Check sheet for the drawn part. Datum: minimum x, y, z corner. Units: mm. Coordinates: 2 decimals unless noted, no trailing zeros. Write each loop counter-clockwise with the first axis right and the second up, starting at its lowest first coordinate (ties: lowest second). Pieces come first, ordered by that corner, then holes. Notation, with made-up numbers: (23.25, 52.25) -> (60.25, 52.25) arc R29 cw to (60.25, 72.25) -> close; hole circle Ø7 at (-25.5, 27.25). An arc over 180 degrees is marked (long way). Answer in a Markdown table with one row per item. Add a question column.
1. Cross-section at A-A on z = 6. Record the cut outline in (x, y), and give its area (3 significant figures).
2. Scan lines: L1, parallel to Y at x = 112, z = 6.25; L2, parallel to Y at x = 106, z = 0.75; L3, parallel to X at y = 469.5, z = 2.5. Record each from-to range of solid material in increasing order. Write a range as from..to.
3. Depth check by flat-ended pin: P1, Ø6, axis at y = 536.5, z = 5, coming from the -X side. Enter the tip coordinate at first touch or a pass-through.
4. Cross-section at B-B on x = 115. Record the cut outline in (y, z), and give its area (3 significant figures).
5. Cross-section at C-C on x = 197.5. Record the cut outline in (y, z) (3 decimals), and give its area (3 significant figures).
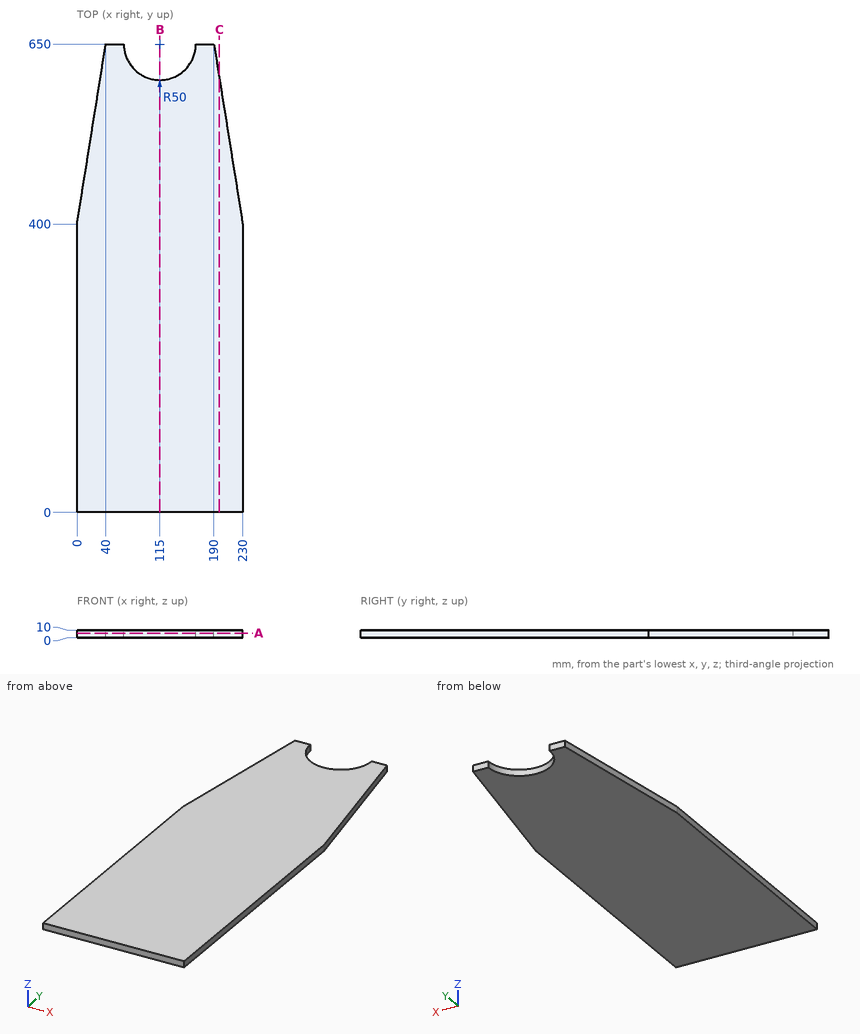
Results found:
| question | item | result |
|---|---|---|
| 1 | outline | (0, 0) -> (230, 0) -> (230, 400) -> (190, 650) -> (165, 650) arc R50 cw to (65, 650) -> (40, 650) -> (0, 400) -> close |
| 1 | area | 136,000 mm^2 |
| 2 | L1 | y = 0..600.09 |
| 2 | L2 | y = 0..600.82 |
| 2 | L3 | x = 11.12..218.88 |
| 3 | P1 | stops at x = 21.36 |
| 4 | outline | (0, 0) -> (600, 0) -> (600, 10) -> (0, 10) -> close |
| 4 | area | 6,000 mm^2 |
| 5 | outline | (0, 0) -> (603.125, 0) -> (603.125, 10) -> (0, 10) -> close |
| 5 | area | 6,030 mm^2 |
